Read the model definition and answer for the solid it produces. Units are mm, in the model's axes. Face numbers are marked on the shaded views. A direction names the side the tool comes from. Round coordinates to 2 decimals unless told otherwise and drop trailing zeros. Order: outer loops, then holes, each group sorted by start corner. A loop starts at its lowest first (then second) coordinate and runs counter-clockwise, first axis right, second up. Notation, with made-up numbers: (-33, -18.75) - (-8, -18.75) arc R21 ccw to (-8, 14.25) - close; hole circle Ø10 at (55.25, -6.75). An arc over 180 degrees is marked (long way). Put each result on its own line as item: value. Start each with the question number.
Q1. Each of these flat-tipped pins is pushed along its axis until it touches: pin 1 Ø5.5 at (y, z) = (15.5, 4.5) entering from -X; pin 2 Ø2 at (x, z) = (-38.5, 9) entering from -Y; pin 3 Ø7 at (x, z) = (-53.69, 0) entering from +Y; pin 4 Ø2.5 at (x, z) = (74.31, 8) entering from +Y. Where does it stop, or does it pass through?
Q2. For a pull along X with two mould halves and no side action, classify the marked faces 1, 2, 3 and 4 as pulls with the +X half, pulls with the -X half, needs draft (parallel to the pull), parting line crosses it, or undercut.
Q3. Which of the six approach directions +Z, -Z, +X, -X, +Y, -Y give full straight-line access (tool end or side, diameter ignored) to the marked faces 5, 6 and 7?
Q4. Section A-A on y = 12 is taken. State how many separate pieces and enclosed holes the cut face has, then the cut area to 3 significant figures.
Q5. Find the intervals of material crossed by line 1 along Y through (x, z) = (22.5, 8.25); line 2 along X through (y, z) = (8.5, -1.5); line 3 along Y through (x, z) = (5, 1.5), in increasing order. Write a range as from..to.
Q6. Section B-B on x = 18 is taken. Give the vertices of the cut face in (y, z).
Q7. Section D-D on x = 41.5 is taken. Give the vertices of the cut face in (y, z).
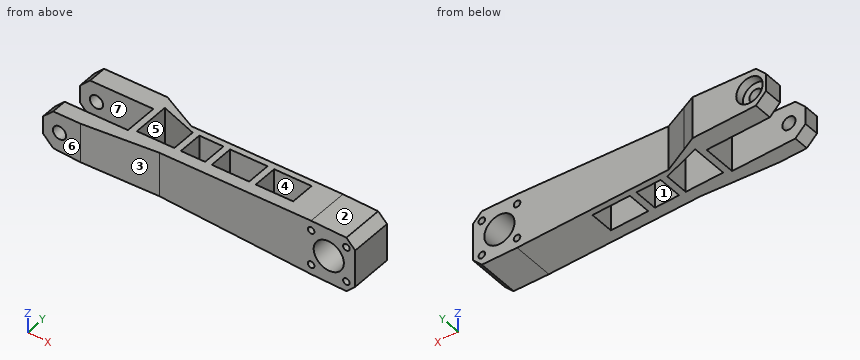
from build123d import *

# Parameters (mm, degrees)
SKETCH1_R           = 1.5
SKETCH1_R_2         = 7.8
SKETCH1_R_3         = 6
SKETCH1_R_4         = 6.85
SKETCH1_R_5         = 3
BOSS_EXTRUDE1_DEPTH = 30.5
CUT_EXTRUDE1_START  = 30.5
SKETCH1_3_R         = 6
CUT_EXTRUDE1_DEPTH  = 3.9
SKETCH1_4_R         = 7.8
CUT_EXTRUDE2_DEPTH  = 0.75
CUT_EXTRUDE3_START  = 30.5
SKETCH1_5_R         = 7.8
CUT_EXTRUDE3_DEPTH  = 1.5
SKETCH3_W           = 33.329175537
SKETCH3_H           = 8.35
SKETCH3_H_2         = 6.85
CUT_EXTRUDE4_DEPTH  = 25
SKETCH4_W           = 11
SKETCH4_H           = 11
CUT_EXTRUDE5_DEPTH  = 25
CUT_EXTRUDE6_START  = 20
SKETCH4_3_W         = 17
SKETCH4_3_H         = 11
CUT_EXTRUDE6_DEPTH  = 30


with BuildPart() as part:
    # Sketch1 → Boss-Extrude1 (new body)
    # profile 1 of 3: a face of its own
    with BuildSketch(Plane(origin=(0, 0, 0), x_dir=(1, 0, 0), z_dir=(0, 1, 0))):
        Polygon((-61.186021101, 4), (-56.589827024, 8.596194078), (58.311754517, 12.502224382), (74.311754517, 12.502224382), (78.313978899, 8.5), (78.313978899, -8.5), (74.311754517, -12.502224382), (58.311754517, -12.502224382), (-56.589827024, -8.596194078), (-61.186021101, -4), align=None)
        with Locations(Location((58.313978899, 8, 0), (0, 0, 90))):
            Circle(SKETCH1_R, mode=Mode.SUBTRACT)
        with Locations(Location((74.313978899, -8, 0), (0, 0, 90))):
            Circle(SKETCH1_R, mode=Mode.SUBTRACT)
        with Locations(Location((58.313978899, -8, 0), (0, 0, 90))):
            Circle(SKETCH1_R, mode=Mode.SUBTRACT)
        with Locations(Location((74.313978899, 8, 0), (0, 0, 90))):
            Circle(SKETCH1_R, mode=Mode.SUBTRACT)
        with Locations((66.313978899, 0)):
            Circle(SKETCH1_R_2, mode=Mode.SUBTRACT)
        with Locations((-53.686021101, 0)):
            Circle(SKETCH1_R_3, mode=Mode.SUBTRACT)
    # profile 2 of 3: a face of its own
    with BuildSketch(Plane(origin=(0, 0, 0), x_dir=(1, 0, 0), z_dir=(0, 1, 0))):
        with Locations((66.313978899, 0)):
            Circle(SKETCH1_R_2)
        with Locations(Location((66.313978899, 0, 0), (0, 0, 90))):
            Circle(SKETCH1_R_4, mode=Mode.SUBTRACT)
    # profile 3 of 3: a face of its own
    with BuildSketch(Plane(origin=(0, 0, 0), x_dir=(1, 0, 0), z_dir=(0, 1, 0))):
        with Locations((-53.686021101, 0)):
            Circle(SKETCH1_R_3)
        with Locations(Location((-53.686021101, 0, 0), (0, 0, 90))):
            Circle(SKETCH1_R_5, mode=Mode.SUBTRACT)
    extrude(amount=BOSS_EXTRUDE1_DEPTH)

    # Sketch1_3 → Cut-Extrude1 (cut)
    with BuildSketch(Plane(origin=(0, 0, 0), x_dir=(1, 0, 0), z_dir=(0, 1, 0)).offset(CUT_EXTRUDE1_START)):
        with Locations(Location((-53.686021101, 0, 0), (0, 0, 270))):
            Circle(SKETCH1_3_R)
    extrude(amount=-CUT_EXTRUDE1_DEPTH, mode=Mode.SUBTRACT)

    # Sketch1_4 → Cut-Extrude2 (cut, symmetric)
    with BuildSketch(Plane(origin=(0, 0, 0), x_dir=(1, 0, 0), z_dir=(0, 1, 0))):
        with Locations(Location((66.313978899, 0, 0), (0, 0, 270))):
            Circle(SKETCH1_4_R)
    extrude(amount=CUT_EXTRUDE2_DEPTH, both=True, mode=Mode.SUBTRACT)

    # Sketch1_5 → Cut-Extrude3 (cut)
    with BuildSketch(Plane(origin=(0, 0, 0), x_dir=(1, 0, 0), z_dir=(0, 1, 0)).offset(CUT_EXTRUDE3_START)):
        with Locations(Location((66.313978899, 0, 0), (0, 0, 270))):
            Circle(SKETCH1_5_R)
    extrude(amount=-CUT_EXTRUDE3_DEPTH, mode=Mode.SUBTRACT)

    # Sketch3 → Cut-Extrude4 (cut, symmetric)
    with BuildSketch(Plane.XY):
        with Locations((-44.521433333, 11.075)):
            Rectangle(SKETCH3_W, SKETCH3_H)
        with Locations((-44.521433333, 18.675)):
            Rectangle(SKETCH3_W, SKETCH3_H_2)
        Polygon((9.374237964, -19.733731398), (78.313978899, 0), (78.313978899, 3), (-10.526021101, 2.935632814), (-44.080457712, 0), align=None)
        Polygon((-10.526021101, 22), (78.313978899, 22), (78.313978899, 30.5), (39.447370773, 56.936233567), (-27.786021101, 30.5), (-21.817807348, 27.528259132), align=None)
    extrude(amount=CUT_EXTRUDE4_DEPTH, both=True, mode=Mode.SUBTRACT)

    # Sketch4 → Cut-Extrude5 (cut, symmetric)
    with BuildSketch(Plane.XY):
        Polygon((-7.856845564, 8.276006159), (-24.856845564, 8.276006159), (-24.856845564, 24.991492085), (-7.856845564, 19.276006159), align=None)
        with Locations((0.643154436, 13.776006159)):
            Rectangle(SKETCH4_W, SKETCH4_H)
        Polygon((9.143154436, 19.276006159), (10.466546433, 19.276006159), (26.143154436, 19.276006159), (26.143154436, 8.276006159), (9.143154436, 8.276006159), align=None)
    extrude(amount=CUT_EXTRUDE5_DEPTH, both=True, mode=Mode.SUBTRACT)

    # Sketch4_3 → Cut-Extrude6 (cut)
    with BuildSketch(Plane.XY.offset(CUT_EXTRUDE6_START)):
        with Locations((37.643154436, 13.776006159)):
            Rectangle(SKETCH4_3_W, SKETCH4_3_H)
    extrude(amount=-CUT_EXTRUDE6_DEPTH, mode=Mode.SUBTRACT)


solid = part.part
Findings:
1. pin 1: x = -27.86
1. pin 2: y = 0.4
1. pin 3: y = 26.6
1. pin 4: through
2. face 1: undercut
2. face 2: needs draft
2. face 3: pulls with the +X half
2. face 4: undercut
3. face 5: +Z, -Z
3. face 6: +Z, -Z, +X, -X, -Y
3. face 7: +Z, -Z, -X
4. separate pieces: 4
4. enclosed holes: 5
4. area: 891 mm2
5. line 1: 2.96..8.28, 19.28..22
5. line 2: -27.86..-24.86, -7.86..-4.86, 6.14..9.14, 26.14..29.14, 46.14..59.63, 73..78.31
5. line 3: 2.95..8.28, 19.28..22
6. outline: (2.96, -11.13) - (8.28, -11.13) - (8.28, 11.13) - (2.96, 11.13) - close; (19.28, -11.13) - (22, -11.13) - (22, 11.13) - (19.28, 11.13) - close
7. outline: (2.97, -11.93) - (22, -11.93) - (22, 11.93) - (19.28, 11.93) - (19.28, -10) - (8.28, -10) - (8.28, 11.93) - (2.97, 11.93) - close
